The listing builds one solid part. Answer for the finished solid, in the listing's coordinates (mm). A direction names the side the tool comes from. Coordinates: 2 decimals unless noted, no trailing zeros. Order: outer loops, then holes, each group sorted by start corner. A loop starts at its lowest first (then second) coordinate and runs counter-clockwise, first axis right, second up. Notation, with made-up numbers: (86.25, -15) -> (132.25, -15) arc R6 cw to (132.25, -10) -> close; hole circle Ø6 at (84.5, -39.5). An arc over 180 degrees is marked (long way). Return JSON: item names as keys, results as strings.
```python
from build123d import *

# Parameters (mm, degrees)
F0_W    = 3
F0_H    = 20.235256
F2_SIZE = 1.5
F3_SIZE = 2


with BuildPart() as f1:
    # F0 (on Front) → F1 (revolve)
    with BuildSketch(Plane.XZ):
        with BuildLine():
            Line((0, 3), (0, 0))
            Line((0, 0), (45, 0))
            Line((45, 0), (45, 3))
            Line((45, 3), (33.75, 3))
            ThreePointArc((33.75, 3), (33, 2.25), (32.25, 3))
            Line((32.25, 3), (3, 3))
            Line((3, 3), (0, 3))
        make_face()
        with Locations((1.5, 13.117628)):
            Rectangle(F0_W, F0_H)
    revolve(axis=Axis((0, 0, 18.496849), (0, 0, 1)))

    # F2
    f2_edges = [f1.edges().sort_by_distance(p)[0] for p in [
        (-45, 0, 3),
    ]]
    chamfer(f2_edges, length=F2_SIZE)

    # F3
    f3_edges = [f1.edges().sort_by_distance(p)[0] for p in [
        (-3, 0, 3),
    ]]
    chamfer(f3_edges, length=F3_SIZE)


solid = f1.part
```
Item 1: Find the intervals of material crossed by probe 1 along Z at (x, y) = (-3, 39.5); probe 2 along Z at (x, y) = (-18.5, -28); probe 3 along Y at (x, z) = (1.5, 4.25), in increasing order.
Answer list:
{"probe 1": "0 to 3", "probe 2": "0 to 2.5", "probe 3": "-3.44 to 3.44"}
Item 2: The part is cut by section A-A on y = 0. Determine the outline of the cut face in (x, z), plus the area to 3 significant figures.
Answer list:
{"outline": "(-45, 0) -> (45, 0) -> (45, 1.5) -> (43.5, 3) -> (33.75, 3) arc R0.75 cw to (32.25, 3) -> (5, 3) -> (3, 5) -> (3, 23.24) -> (-3, 23.24) -> (-3, 5) -> (-5, 3) -> (-32.25, 3) arc R0.75 cw to (-33.75, 3) -> (-43.5, 3) -> (-45, 1.5) -> close", "area": "391 mm2"}
Item 3: Flat-ended cylindrical pins translate along their axes: pin 1 (4 mm diameter, centred on y = -34.5, z = 3, fed in from +X); pin 2 (12 mm diameter, centred on x = -3.5, z = 20.5, fed in from -Y); pin 3 (8 mm diameter, centred on y = -21.5, z = 6.5, fed in from +X). Find the tip coordinate at first contact, or state that the pin passes through.
Answer list:
{"pin 1": "x = 30.4", "pin 2": "y = -3", "pin 3": "x = 38.87"}
Item 4: The part is cut by section B-B on z = 16.25. Determine the outline of the cut face in (x, y).
Answer list:
{"outline": "circle Ø6 at (0, 0)"}
Item 5: Which of the six approach directions +Z, -Z, +X, -X, +Y, -Y give full straight-line access (tool end or side, diameter ignored) to faces 1 (the cylindrical face through (20.765, -39.923, 0.76)), 2 (the cylindrical face through (-3, 0, 14))?
Answer list:
{"face 1": "+Z, -Z", "face 2": "+Z"}
